```python
from build123d import *

# Parameters (mm, degrees)
F1_DEPTH = 71.12
F2_DEPTH = 87.376
F3_ANGLE = 275


with BuildPart() as f1:
    # F0 (on Front) → F1 (new body)
    with BuildSketch(Plane.XZ):
        with BuildLine():
            Line((-129.7797858715, 33.2981981337), (-129.7797858715, -36.6309396923))
            Line((-129.7797858715, -36.6309396923), (10.8276167884, -36.6309396923))
            ThreePointArc((10.8276167884, -36.6309396923), (23.7625826148, -24.1752902471), (16.6507605463, -7.686550729))
            Line((16.6507605463, -7.686550729), (-49.0343049169, 33.2981981337))
            Line((-49.0343049169, 33.2981981337), (-129.7797858715, 33.2981981337))
        make_face()
    extrude(amount=F1_DEPTH)

    # F2 (add): a face of the model
    f2_faces = [f1.faces().sort_by_distance(p)[0] for p in [
        (-89.4070453942, -35.56, 33.2981981337),
    ]]
    extrude(f2_faces, amount=F2_DEPTH)

    # F2_face (on face) → F3 (revolve)
    with BuildSketch(Plane(origin=(-74.6235346517, -71.12, 30.893227171), x_dir=(1, 0, 0), z_dir=(0, -1, 0))):
        with BuildLine():
            Line((91.274295198, -38.5797779), (25.5892297349, 2.4049709627))
            Line((25.5892297349, 2.4049709627), (25.5892297349, 89.7809709627))
            Line((25.5892297349, 89.7809709627), (-55.1562512198, 89.7809709627))
            Line((-55.1562512198, 89.7809709627), (-55.1562512198, -67.5241668633))
            Line((-55.1562512198, -67.5241668633), (85.4511514402, -67.5241668633))
            ThreePointArc((85.4511514402, -67.5241668633), (98.3861172665, -55.0685174181), (91.274295198, -38.5797779))
        make_face()
    revolve(axis=Axis((-129.7797858715, -71.12, 42.0216292207), (0, 0, -1)), revolution_arc=F3_ANGLE)


solid = f1.part
```
Check sheet for the modelled part. Datum: model origin and axes. Units: mm. A direction names the side the tool comes from. Round coordinates to 2 decimals unless told otherwise and drop trailing zeros. Order: outer loops, then holes, each group sorted by start corner. A loop starts at its lowest first (then second) coordinate and runs counter-clockwise, first axis right, second up.
1) Section check A-A (z = 97). Record the boundary of the cut face in (x, y).
2) Scan lines: line 1 (Z direction, x = -154, y = 45); line 2 (X direction, y = -53.5, z = 88); line 3 (Z direction, x = -209, y = -54). Record each from-to range of solid material in increasing order.
3) Go/stop test with flat-tipped pins: pin 1 Ø1 at (x, z) = (-172.5, 20) entering from +Y; pin 2 Ø5 at (x, z) = (-178, 87) entering from -Y; pin 3 Ø21.5 at (y, z) = (-20, 88.5) entering from +X. Record where each tip stops, or that it passes through.
4) Section check B-B (z = -3). Record the boundary of the cut face in (x, y).
5) Mould release check, pull along Y, two halves, no side actions. Record for faces 4 (the flat face through (-121.046, 28.712, 1.606)), 5 (the conical face through (-189.72, -129.87, 31.31)), 6 (the cylindrical face through (23.708, -35.062, -24.437)): +Y half, -Y half, draft (parallel to the pull), parting line (faces both ways), or undercut.
6) Tool access check on faces 1 (the flat face through (-49.034, -35, 76)), 2 (the flat face through (-131, -72, 120.674)), 3 (the cylindrical face through (-187.446, -127.64, 77.598)). Record the directions out of +Z, -Z, +X, -X, +Y, -Y that give a thin tool (end or side, any length) a straight path to the whole face; none if there is none.
Result:
1. outline: (-123.56, 0) - (-122.74, 9.32) arc R80.75 ccw (long way) to (-49.03, -71.12) - (-49.03, 0) - close
2. line 1: z = -36.63 to 9.67
2. line 2: x = -208.58 to -49.03
2. line 3: z = -36.63 to 33.11
3. pin 1: stops at y = 22.48
3. pin 2: stops at y = -137.67
3. pin 3: stops at x = -49.03
4. outline: (-123.56, 0) - (-117.67, 67.27) arc R138.92 ccw (long way) to (9.14, -71.12) - (9.14, 0) - close
5. face 4: undercut
5. face 5: parting line
5. face 6: draft
6. face 1: +Z, +X, +Y, -Y
6. face 2: +Z, +X, -X, +Y, -Y
6. face 3: +Z
